Geometry check sheet. Reference: the model listing, model coordinates, mm. Give positions to 0.01 mm unless a question says otherwise; leave off trailing zeros.
1. Cross-section at A-A, the plane x = 0. State how many separate pieces and enclosed holes the cut face has, plus the area to 3 significant figures.
2. Release check for a two-part mould opening along X. For faces 1 (the cylindrical face through (-6.88, -48.28, 2.06)), 2 (the flat face through (-9, -98.712, 2)), 3 (the flat face through (28.275, 0, 2)) record: +X half, -X half, draft (parallel to the pull), parting line (faces both ways), or undercut.
3. Material ranges on L1, parallel to X at y = 52, z = 1.7 (3 decimals); L2, parallel to X at y = -60, z = 3.55 (3 decimals), recorded low to high.
from build123d import *

# Parameters (mm, degrees)
BOSS_EXTRUDE1_OUTLINE_W                         = 56.55
BOSS_EXTRUDE1_OUTLINE_H                         = 197.425
BOSS_EXTRUDE1_DEPTH                             = 4.064
SKETCH4_R                                       = 5
CUT_EXTRUDE2_DEPTH                              = 103.762587439
LPATTERN3_COUNT                                 = 13
LPATTERN3_PITCH                                 = 11
SKETCH5_W                                       = 4.064
SKETCH5_H                                       = 197.425
BOSS_EXTRUDE2_DEPTH                             = 19.525
SKETCH14_W                                      = 76.075
SKETCH14_H                                      = 4.064
BOSS_EXTRUDE3_DEPTH                             = 3.175
M4_CLEARANCE_HOLE1_D                            = 4.5
CSK_FOR_M3_FLAT_HEAD_MACHINE_SCREW2_D           = 3.4
CSK_FOR_M3_FLAT_HEAD_MACHINE_SCREW2_CSINK_D     = 6.3
CSK_FOR_M3_FLAT_HEAD_MACHINE_SCREW2_CSINK_ANGLE = 90


# Read off the part's stored shape, not the designer's step: Boss-Extrude1
with BuildPart() as part:
    # Boss-Extrude1 outline → Boss-Extrude1 (new body)
    with BuildSketch(Plane.XY):
        Rectangle(BOSS_EXTRUDE1_OUTLINE_W, BOSS_EXTRUDE1_OUTLINE_H)
    extrude(amount=BOSS_EXTRUDE1_DEPTH)

    # Sketch4 → Cut-Extrude2 (cut, through all)
    with BuildSketch(Plane.XY.offset(4.064)):
        with Locations((0, -57.369162839)):
            Circle(SKETCH4_R)
        with Locations((11.5, -57.369162839)):
            Circle(SKETCH4_R)
        with Locations((-11.5, -57.369162839)):
            Circle(SKETCH4_R)
    cut_extrude2 = extrude(amount=-CUT_EXTRUDE2_DEPTH, mode=Mode.SUBTRACT)

    # LPattern3: Cut-Extrude2 ×13
    with Locations(*[(0, i * LPATTERN3_PITCH, 0) for i in range(1, LPATTERN3_COUNT)]):
        add(cut_extrude2, mode=Mode.SUBTRACT)

    # Sketch5 → Boss-Extrude2 (add)
    with BuildSketch(Plane.ZY.offset(28.275)):
        with Locations((2.032, 0)):
            Rectangle(SKETCH5_W, SKETCH5_H)
    extrude(amount=BOSS_EXTRUDE2_DEPTH)

    # Sketch14 → Boss-Extrude3 (add)
    with BuildSketch(Plane(origin=(0, 98.7125, 0), x_dir=(1, 0, 0), z_dir=(0, 1, 0))):
        with Locations((-9.7625, -2.032)):
            Rectangle(SKETCH14_W, SKETCH14_H)
    extrude(amount=BOSS_EXTRUDE3_DEPTH)

    # M4 Clearance Hole1 (through all)
    with Locations(Plane.XY.offset(4.064)):
        with Locations((0, 92.3625001), (0, -78.8874999)):
            Hole(M4_CLEARANCE_HOLE1_D / 2)

    # CSK for M3 Flat Head Machine Screw2 (through all)
    with Locations(Plane(origin=(0, 0, 0), x_dir=(-1, 0, 0), z_dir=(0, 0, -1))):
        with Locations((17.4625, -78.8874999), (-17.4625, 92.3625001)):
            CounterSinkHole(CSK_FOR_M3_FLAT_HEAD_MACHINE_SCREW2_D / 2, CSK_FOR_M3_FLAT_HEAD_MACHINE_SCREW2_CSINK_D / 2, counter_sink_angle=CSK_FOR_M3_FLAT_HEAD_MACHINE_SCREW2_CSINK_ANGLE)


solid = part.part
Result:
1. separate pieces: 16
1. enclosed holes: 0
1. area: 250 mm2
2. face 1: undercut
2. face 2: draft
2. face 3: +X half
3. L1: x = -47.8 to -16.46, -6.54 to -4.96, 4.96 to 6.54, 16.46 to 28.275
3. L2: x = -47.8 to -15.752, -7.248 to -4.252, 4.252 to 7.248, 15.752 to 28.275
